Could you check a few things on this model? Use its own coordinates, in mm. A direction names the side the tool comes from. Give positions to 0.01 mm unless a question says otherwise; leave off trailing zeros. Write each loop counter-clockwise with the first axis right and the second up, starting at its lowest first coordinate (ties: lowest second). Pieces come first, ordered by that corner, then holes. Notation, with made-up numbers: M 63.25,88.25 L 73.25,88.25 A13 cw 73.25,99.25 Z; hole C 29.25,86.5 d11. An arc over 180 degrees is marked long. Answer as a JSON object with one key per item and string values. Group by question number.
```python
from build123d import *

# Parameters (mm, degrees)
SKETCH1_W           = 99.30160125
SKETCH1_H           = 60.173202502
BOSS_EXTRUDE1_DEPTH = 29.21
SKETCH1_23_W        = 99.30160125
SKETCH1_23_H        = 60.173202502
BOSS_EXTRUDE2_DEPTH = 2.54
CUT_EXTRUDE1_START  = 29.21
SKETCH1_25_R        = 2.413
CUT_EXTRUDE1_DEPTH  = 12.192
SKETCH1_28_R        = 1.651
BOSS_EXTRUDE5_DEPTH = 10.16
SKETCH6_W           = 8.89
SKETCH6_H           = 10.668
CUT_EXTRUDE2_DEPTH  = 10.16
SKETCH8_W           = 16.51
SKETCH8_H           = 11.43
CUT_EXTRUDE4_DEPTH  = 10.16
SKETCH10_R          = 2.032
CUT_EXTRUDE7_DEPTH  = 6.200800625
REVOLVE1_ANGLE      = 180
REVOLVE2_ANGLE      = 180
SKETCH13_R          = 0.45
CUT_EXTRUDE8_DEPTH  = 7.62
FILLET2_R           = 2.54


with BuildPart() as part:
    # Sketch1 → Boss-Extrude1 (new body)
    with BuildSketch(Plane(origin=(0, 0, 0), x_dir=(1, 0, 0), z_dir=(0, 1, 0))):
        Rectangle(SKETCH1_W, SKETCH1_H)
        with BuildLine():
            ThreePointArc((-44.45, 19.685), (-40.77247861, 21.208279236), (-39.249199375, 24.885800625))
            Line((-39.249199375, 24.885800625), (39.249199375, 24.885800625))
            ThreePointArc((39.249199375, 24.885800625), (40.77247861, 21.208279236), (44.45, 19.685))
            Line((44.45, 19.685), (44.45, -24.885800625))
            Line((44.45, -24.885800625), (-39.249199375, -24.885800625))
            ThreePointArc((-39.249199375, -24.885800625), (-40.77247861, -21.208279236), (-44.45, -19.685))
            Line((-44.45, -19.685), (-44.45, 19.685))
        make_face(mode=Mode.SUBTRACT)
    extrude(amount=BOSS_EXTRUDE1_DEPTH)

    # Sketch1<23> → Boss-Extrude2 (add)
    with BuildSketch(Plane(origin=(0, 0, 0), x_dir=(1, 0, 0), z_dir=(0, 1, 0))):
        Rectangle(SKETCH1_23_W, SKETCH1_23_H)
    extrude(amount=-BOSS_EXTRUDE2_DEPTH)

    # Sketch1<25> → Cut-Extrude1 (cut)
    with BuildSketch(Plane(origin=(0, 0, 0), x_dir=(1, 0, 0), z_dir=(0, 1, 0)).offset(CUT_EXTRUDE1_START)):
        with Locations((-44.45, 24.885800625)):
            Circle(SKETCH1_25_R)
        with Locations((44.45, 24.885800625)):
            Circle(SKETCH1_25_R)
        with Locations((-44.45, -24.885800625)):
            Circle(SKETCH1_25_R)
    extrude(amount=-CUT_EXTRUDE1_DEPTH, mode=Mode.SUBTRACT)

    # Sketch1<28> → Boss-Extrude5 (add)
    with BuildSketch(Plane(origin=(0, 0, 0), x_dir=(1, 0, 0), z_dir=(0, 1, 0))):
        with Locations((42.186757457, 17.024199375)):
            Circle(SKETCH1_28_R)
        with Locations((-36.852757457, -22.225)):
            Circle(SKETCH1_28_R)
        with Locations((-36.852757457, 17.024199375)):
            Circle(SKETCH1_28_R)
        with Locations((42.186757457, -22.225)):
            Circle(SKETCH1_28_R)
    extrude(amount=BOSS_EXTRUDE5_DEPTH)

    # Sketch6 → Cut-Extrude2 (cut)
    with BuildSketch(Plane(origin=(0, 0, 24.885800625), x_dir=(-1, 0, 0), z_dir=(0, 0, -1))):
        with Locations((-29.845, 11.684)):
            Rectangle(SKETCH6_W, SKETCH6_H)
    extrude(amount=-CUT_EXTRUDE2_DEPTH, mode=Mode.SUBTRACT)

    # Sketch8 → Cut-Extrude4 (cut)
    with BuildSketch(Plane.XY.offset(30.086601251)):
        with Locations((12.573, 13.589)):
            Rectangle(SKETCH8_W, SKETCH8_H)
    extrude(amount=-CUT_EXTRUDE4_DEPTH, mode=Mode.SUBTRACT)

    # Sketch10 → Cut-Extrude7 (cut, through all)
    with BuildSketch(Plane.ZY.offset(-44.45)):
        with Locations((17.265800625, 9.5758)):
            Circle(SKETCH10_R)
        with Locations((5.835800625, 9.5758)):
            Circle(SKETCH10_R)
    extrude(amount=-CUT_EXTRUDE7_DEPTH, mode=Mode.SUBTRACT)

    # Sketch12 → Revolve1 (revolve)
    with BuildSketch(Plane(origin=(49.650800625, 0, 0), x_dir=(0, 0, -1), z_dir=(1, 0, 0))):
        with BuildLine():
            Line((-17.265800625, 11.6078), (-17.265800625, 12.1158))
            ThreePointArc((-17.265800625, 12.1158), (-19.805800625, 9.5758), (-17.265800625, 7.0358))
            Line((-17.265800625, 7.0358), (-17.265800625, 7.5438))
            ThreePointArc((-17.265800625, 7.5438), (-19.297800625, 9.5758), (-17.265800625, 11.6078))
        make_face()
    revolve(axis=Axis((49.650800625, 12.1158, 17.265800625), (0, 1, 0)), revolution_arc=REVOLVE1_ANGLE)

    # Sketch12<4> → Revolve2 (revolve)
    with BuildSketch(Plane(origin=(49.650800625, 0, 0), x_dir=(0, 0, -1), z_dir=(1, 0, 0))):
        with BuildLine():
            ThreePointArc((-5.835800625, 7.0358), (-3.295800625, 9.5758), (-5.835800625, 12.1158))
            Line((-5.835800625, 12.1158), (-5.835800625, 11.6078))
            ThreePointArc((-5.835800625, 11.6078), (-3.803800625, 9.5758), (-5.835800625, 7.5438))
            Line((-5.835800625, 7.5438), (-5.835800625, 7.0358))
        make_face()
    revolve(axis=Axis((49.650800625, 12.1158, 5.835800625), (0, -1, 0)), revolution_arc=REVOLVE2_ANGLE)

    # Sketch13 → Cut-Extrude8 (cut)
    with BuildSketch(Plane(origin=(49.650800625, 0, 0), x_dir=(0, 0, -1), z_dir=(1, 0, 0))):
        with Locations((-18.789800625, 24.384)):
            Circle(SKETCH13_R)
        with Locations((-15.741800625, 24.384)):
            Circle(SKETCH13_R)
    extrude(amount=-CUT_EXTRUDE8_DEPTH, mode=Mode.SUBTRACT)

    # Fillet2
    fillet2_edges = [part.edges().sort_by_distance(p)[0] for p in [
        (-49.650800625, 13.335, -30.086601251),
        (49.650800625, 13.335, -30.086601251),
        (49.650800625, 13.335, 30.086601251),
        (-49.650800625, 13.335, 30.086601251),
    ]]
    fillet(fillet2_edges, radius=FILLET2_R)


solid = part.part
```
1) If we section it at D-D, the plane x = 1: List the corners of the cut face in (y, z) for me.
2) We'd pull the mould along Z, two halves only. Please class faces 1 (the cylindrical face through (-40.81, 14.4, -21.17)), 2 (the cylindrical face through (-48.89, 13.56, 29.36)), 3 (the cylindrical face through (47.01, 7.77, 6.77)), 4 (the flat face through (30, 6.35, 27)): released by +Z, released by -Z, zero draft, split by the parting line, or undercut.
3) If we section it at C-C, the plane z = -13: List the corners of the cut face in (x, y) for me, plus the area to 3 significant figures.
4) Please list where these lines run through material, in increasing order: line 1 along Z through (x, y) = (35.5, 8.5); line 2 along X through (y, z) = (6.5, 15); line 3 along Z through (x, y) = (44, 26). Write a range as from..to.
5) I'm going to push flat-ended pins straight in: pin 1 (2 mm diameter, centred on y = 18, z = 23, fed in from +X); pin 2 (3.5 mm diameter, centred on x = -37.5, z = 22, fed in from +Y); pin 3 (15 mm diameter, centred on x = -8, z = 12.5, fed in from +Y). Where does each tip first touch, or does it pass through?
6) If we section it at A-A, the plane y = 1.5: List the corners of the cut face in (x, z) for me (3 decimals).
7) If we section it at B-B, the plane x = 15.5: List the corners of the cut face in (y, z) for me.
8) For faces 5 (the flat face through (20.828, 14, 28)), 6 (the flat face through (-1, 14, 30.087)), 7 (the flat face through (-44.45, 14, 0)), which set-ups out of +Z, -Z, +X, -X, +Y, -Y let a thin tool reach every point of the face, with its end or its side?
Taken from the geometry:
{
 "1": {"outline": "M -2.54,-30.09 L 29.21,-30.09 L 29.21,-24.89 L 0,-24.89 L 0,24.89 L 29.21,24.89 L 29.21,30.09 L -2.54,30.09 Z"},
 "2": {"face 1": "undercut", "face 2": "released by +Z", "face 3": "undercut", "face 4": "zero draft"},
 "3": {"outline": "M -49.65,-2.54 L 49.65,-2.54 L 49.65,29.21 L 44.45,29.21 L 44.45,0 L -44.45,0 L -44.45,29.21 L -49.65,29.21 Z", "area": "556 mm²"},
 "4": {"line 1": "-30.09..-24.89, 24.89..30.09", "line 2": "-49.65..-44.45, 44.45..49.65", "line 3": "-30.09..-27.26, -22.52..-19.7, 24.89..30.09"},
 "5": {"pin 1": "x = 49.65", "pin 2": "y = 10.16", "pin 3": "y = 0"},
 "6": {"outline": "M -49.651,-27.547 A2.54 ccw -47.111,-30.087 L 47.111,-30.087 A2.54 ccw 49.651,-27.547 L 49.651,27.547 A2.54 ccw 47.111,30.087 L -47.111,30.087 A2.54 ccw -49.651,27.547 Z; C -36.853,-17.024 d3.302; C -36.853,22.225 d3.302; C 42.187,-17.024 d3.302; C 42.187,22.225 d3.302; hole M -44.45,-19.685 A5.201 cw -39.249,-24.886 L 39.249,-24.886 A5.201 cw 44.45,-19.685 L 44.45,24.886 L -39.249,24.886 A5.201 cw -44.45,19.685 Z"},
 "7": {"outline": "M -2.54,-30.09 L 29.21,-30.09 L 29.21,-24.89 L 0,-24.89 L 0,24.89 L 7.87,24.89 L 7.87,30.09 L -2.54,30.09 Z; M 19.3,24.89 L 29.21,24.89 L 29.21,30.09 L 19.3,30.09 Z"},
 "8": {"face 5": "+Z", "face 6": "+Z, +X, -X, +Y, -Y", "face 7": "+Y"}
}
